from build123d import *

# Parameters (mm, degrees)
F0_W     = 762
F0_H     = 584.2
F1_DEPTH = 254
F3_DEPTH = 247.65
F5_DEPTH = 254
F6_DEPTH = 254
F7_DEPTH = 247.65


with BuildPart() as f1:
    # F0 (on Top) → F1 (new body)
    with BuildSketch(Plane.XY):
        with Locations((3.6051012576, 23.4938759938)):
            Rectangle(F0_W, F0_H)
    extrude(amount=F1_DEPTH)

    # F2 (on face) → F3 (cut)
    with BuildSketch(Plane.XY.offset(254)):
        Polygon((-371.0448987424, 309.2438759938), (-371.0448987424, 295.6585884094), (-371.0448987424, 213.9938759938), (378.2551012576, 213.9938759938), (378.2551012576, 277.7049839497), (378.2551012576, 309.2438759938), align=None)
    extrude(amount=-F3_DEPTH, mode=Mode.SUBTRACT)

    # F4 (on face) → F5 (join)
    with BuildSketch(Plane.XY.offset(254)):
        Polygon((384.6051012576, 315.5938759938), (384.6051012576, 175.8938759938), (384.6051012576, -40.0061240062), (384.6051012576, -52.7061240062), (384.6051012576, -268.6061240062), (390.9551012576, -268.6061240062), (390.9551012576, 315.5938759938), align=None)
    extrude(amount=-F5_DEPTH)

    # F4 (on face) → F6 (join)
    with BuildSketch(Plane.XY.offset(254)):
        Polygon((390.9551012576, -268.6061240062), (384.6051012576, -268.6061240062), (263.9551012576, -268.6061240062), (257.6051012576, -268.6061240062), (136.9551012576, -268.6061240062), (130.6051012576, -268.6061240062), (9.9551012576, -268.6061240062), (3.6051012576, -268.6061240062), (-117.0448987424, -268.6061240062), (-123.3948987424, -268.6061240062), (-244.0448987424, -268.6061240062), (-250.3948987424, -268.6061240062), (-371.0448987424, -268.6061240062), (-377.3948987424, -268.6061240062), (-377.3948987424, -274.9561240062), (390.9551012576, -274.9561240062), align=None)
    extrude(amount=-F6_DEPTH)

    # F4 (on face) → F7 (cut)
    with BuildSketch(Plane.XY.offset(254)):
        Polygon((-244.0448987424, -231.7013091296), (-244.0448987424, -268.6061240062), (-123.3948987424, -268.6061240062), (-123.3948987424, -229.8385000676), (-123.3948987424, -52.7061240062), (-244.0448987424, -52.7061240062), align=None)
        Polygon((-117.0448987424, -229.8385000676), (-117.0448987424, -268.6061240062), (3.6051012576, -268.6061240062), (3.6051012576, -232.6196825951), (3.6051012576, -52.7061240062), (-117.0448987424, -52.7061240062), align=None)
        Polygon((9.9551012576, -268.6061240062), (130.6051012576, -268.6061240062), (130.6051012576, -242.5831056088), (130.6051012576, -52.7061240062), (9.9551012576, -52.7061240062), (9.9551012576, -232.6196825951), align=None)
        Polygon((136.9551012576, -268.6061240062), (257.6051012576, -268.6061240062), (257.6051012576, -243.7552756518), (257.6051012576, -52.7061240062), (136.9551012576, -52.7061240062), (136.9551012576, -242.5831056088), align=None)
        Polygon((384.6051012576, -268.6061240062), (384.6051012576, -52.7061240062), (263.9551012576, -52.7061240062), (263.9551012576, -243.7552756518), (263.9551012576, -268.6061240062), align=None)
        Polygon((257.6051012576, 151.0430276394), (257.6051012576, 175.8938759938), (136.9551012576, 175.8938759938), (136.9551012576, 149.8708575964), (136.9551012576, -40.0061240062), (257.6051012576, -40.0061240062), align=None)
        Polygon((130.6051012576, 149.8708575964), (130.6051012576, 175.8938759938), (9.9551012576, 175.8938759938), (9.9551012576, 139.9074345827), (9.9551012576, -40.0061240062), (130.6051012576, -40.0061240062), align=None)
        Polygon((384.6051012576, 175.8938759938), (378.2551012576, 175.8938759938), (263.9551012576, 175.8938759938), (263.9551012576, 151.0430276394), (263.9551012576, -40.0061240062), (384.6051012576, -40.0061240062), align=None)
        Polygon((3.6051012576, 175.8938759938), (-117.0448987424, 175.8938759938), (-117.0448987424, 137.1262520552), (-117.0448987424, -40.0061240062), (3.6051012576, -40.0061240062), (3.6051012576, 139.9074345827), align=None)
        Polygon((-123.3948987424, 175.8938759938), (-244.0448987424, 175.8938759938), (-244.0448987424, 138.9890611172), (-244.0448987424, -40.0061240062), (-123.3948987424, -40.0061240062), (-123.3948987424, 137.1262520552), align=None)
        Polygon((-250.3948987424, 175.8938759938), (-371.0448987424, 175.8938759938), (-371.0448987424, -40.0061240062), (-342.720925808, -40.0061240062), (-250.3948987424, -40.0061240062), (-250.3948987424, 138.9890611172), align=None)
        Polygon((-371.0448987424, -52.7061240062), (-371.0448987424, -268.6061240062), (-250.3948987424, -268.6061240062), (-250.3948987424, -231.7013091296), (-250.3948987424, -52.7061240062), align=None)
    extrude(amount=-F7_DEPTH, mode=Mode.SUBTRACT)


solid = f1.part
Here's how the part is built. I have some questions about the finished solid (model axes, mm). A direction names the side the tool comes from. Give positions to 0.01 mm unless a question says otherwise; leave off trailing zeros. Order: outer loops, then holes, each group sorted by start corner. A loop starts at its lowest first (then second) coordinate and runs counter-clockwise, first axis right, second up. Notation, with made-up numbers: (-19.5, -36) -> (11.5, -36) arc R24 ccw to (11.5, -24) -> close; hole circle Ø8 at (42, 47.5). An arc over 180 degrees is marked (long way). One line per item, written item: value. Start each with the question number.
1. Will this pin go through, and if not, where does the flat tip stop? pin 1 Ø1.5 at (x, y) = (16, -110.5) entering from +Z.
2. We'd pull the mould along X, two halves only. Please class faces 3 (the face through (325, -52.706, 132)), 4 (the face through (-377.395, 24, 129)), 5 (the face through (12, 315.594, 129)): released by +X, released by -X, zero draft, split by the parting line, or undercut.
3. Imagine slicing it at D-D, the plane y = -63. List the corners of the cut face in (x, z) for me, plus the area to 3 significant figures.
4. Imagine slicing it at B-B, the plane x = 208. List the corners of the cut face in (y, z) for me, plus the area to 3 significant figures.
5. For faces 1 (the face through (1, 24, 0)), 2 (the face through (384.605, 66, 132)), which set-ups out of +Z, -Z, +X, -X, +Y, -Y let a thin tool reach every point of the face, with its end or its side?
6. Imagine slicing it at A-A, the plane y = 257. List the corners of the cut face in (x, z) for me.
7. I need wall thicknesses on probe 1 along Y at (x, z) = (96, 142.5); probe 2 along Z at (x, y) = (-47, -123). Which ranges of each line are inside material? Lowest first, please. Write a range as from..to.
8. Imagine slicing it at C-C, the plane z = 75. Count the separate pieces of the cut face and the enclosed holes in it, plus the area to 3 significant figures.
Values follow:
1. pin 1: stops at z = 6.35
2. face 3: undercut
2. face 4: released by -X
2. face 5: zero draft
3. outline: (-377.39, 0) -> (390.96, 0) -> (390.96, 254) -> (384.61, 254) -> (384.61, 6.35) -> (263.96, 6.35) -> (263.96, 254) -> (257.61, 254) -> (257.61, 6.35) -> (136.96, 6.35) -> (136.96, 254) -> (130.61, 254) -> (130.61, 6.35) -> (9.96, 6.35) -> (9.96, 254) -> (3.61, 254) -> (3.61, 6.35) -> (-117.04, 6.35) -> (-117.04, 254) -> (-123.39, 254) -> (-123.39, 6.35) -> (-244.04, 6.35) -> (-244.04, 254) -> (-250.39, 254) -> (-250.39, 6.35) -> (-371.04, 6.35) -> (-371.04, 254) -> (-377.39, 254) -> close
3. area: 15,900 mm2
4. outline: (-274.96, 0) -> (315.59, 0) -> (315.59, 254) -> (309.24, 254) -> (309.24, 6.35) -> (213.99, 6.35) -> (213.99, 254) -> (175.89, 254) -> (175.89, 6.35) -> (-40.01, 6.35) -> (-40.01, 254) -> (-52.71, 254) -> (-52.71, 6.35) -> (-268.61, 6.35) -> (-268.61, 254) -> (-274.96, 254) -> close
4. area: 19,500 mm2
5. face 1: -Z, +X, -X, +Y, -Y
5. face 2: +Z
6. outline: (-377.39, 0) -> (390.96, 0) -> (390.96, 254) -> (378.26, 254) -> (378.26, 6.35) -> (-371.04, 6.35) -> (-371.04, 254) -> (-377.39, 254) -> close
7. probe 1: y = -274.96..-268.61, -52.71..-40.01, 175.89..213.99, 309.24..315.59
7. probe 2: z = 0..6.35
8. separate pieces: 1
8. enclosed holes: 13
8. area: 69,800 mm2
